from build123d import *

# Parameters (mm, degrees)
F1_START = 10
F0_R     = 79.5
F1_DEPTH = 5
F0_R_2   = 82
F2_DEPTH = 15
F0_R_3   = 87.5
F3_DEPTH = 4
F4_SIZE2 = 2.7474774195
F4_SIZE  = 1
F5_SIZE2 = 5.4949548389
F5_SIZE  = 2


with BuildPart() as f1:
    # F0 (on Top) → F1 (new body)
    with BuildSketch(Plane.XY.offset(F1_START)):
        Circle(F0_R)
    extrude(amount=F1_DEPTH)

    # F0 (on Top) → F2 (join)
    with BuildSketch(Plane.XY):
        Circle(F0_R_2)
        Circle(F0_R, mode=Mode.SUBTRACT)
    extrude(amount=F2_DEPTH)

    # F0 (on Top) → F3 (join)
    with BuildSketch(Plane.XY):
        Circle(F0_R_3)
        Circle(F0_R_2, mode=Mode.SUBTRACT)
    extrude(amount=F3_DEPTH)

    # F4
    f4_edges = [f1.edges().sort_by_distance(p)[0] for p in [
        (-82, 0, 15),
    ]]
    f4_side = f1.faces().sort_by_distance((0, 0, 15))[0]
    chamfer(f4_edges, length=F4_SIZE, length2=F4_SIZE2, reference=f4_side)

    # F5
    f5_edges = [f1.edges().sort_by_distance(p)[0] for p in [
        (-79.5, 0, 0),
    ]]
    f5_side = f1.faces().sort_by_distance((-81.974874, 0, 0))[0]
    chamfer(f5_edges, length=F5_SIZE, length2=F5_SIZE2, reference=f5_side)


solid = f1.part
Build history of the part. All positions in model axes, mm. A direction names the side the tool comes from. Round coordinates to 2 decimals unless told otherwise and drop trailing zeros. Write each loop counter-clockwise with the first axis right and the second up, starting at its lowest first coordinate (ties: lowest second). Pieces come first, ordered by that corner, then holes. Notation, with made-up numbers: M 85,82 L 101,82 A32 cw 101,110 Z; hole C 46.25,-4 d6. An arc over 180 degrees is marked long. Answer in a Markdown table with one row per item.
1. Which spindle directions (+Z, -Z, +X, -X, +Y, -Y) get a long thin tool onto all of the face, cutting with end or side? Do faces 5 (the face through (-78, -26, 4)), 6 (the face through (-72, 39, 0)), 7 (the face through (-1, 1, 10)). Say none if no direction does.
Geometry check:
| item | result |
|---|---|
| face 5 | +Z |
| face 6 | -Z, +X, -X, +Y, -Y |
| face 7 | -Z |
2. Saw through at A-A (y = 0). List the corners of the cut face in (x, z), and give its area (3 significant figures).
Geometry check:
| item | result |
|---|---|
| outline | M -87.5,0 L -81.5,0 L -79.5,5.49 L -79.5,10 L 79.5,10 L 79.5,5.49 L 81.5,0 L 87.5,0 L 87.5,4 L 82,4 L 82,12.25 L 81,15 L -81,15 L -82,12.25 L -82,4 L -87.5,4 Z |
| area | 900 mm2 |
3. Flat gauge pins, fed straight in: P1, Ø1, axis at x = 21.5, z = 11, coming from the +Y side; P2, Ø3, axis at x = 43, y = 25.5, coming from the -Z side; P3, Ø3, axis at y = 52.5, z = 12, coming from the +X side. Where does each tip first touch, or does it go through?
Geometry check:
| item | result |
|---|---|
| P1 | y = 79.27 |
| P2 | z = 10 |
| P3 | x = 64.21 |
4. Mould opens along Y. For faces 1 (the face through (-10.349, 78.823, 7.716)), 2 (the face through (-63.17, -48.43, 5.23)), 3 (the face through (77.32, 24.35, 14.83)), 4 (the face through (-1, 1, 15)) say: +Y half, -Y half, draft (parallel to the pull), parting line (faces both ways), or undercut.
Geometry check:
| item | result |
|---|---|
| face 1 | undercut |
| face 2 | undercut |
| face 3 | parting line |
| face 4 | draft |
5. Probe L1, parallel to Y at x = 0, z = 7.1; L2, parallel to Z at x = 71, y = -35; L3, parallel to Y at x = 36.5, z = 5.5. List the from-to ranges inside material, lowest first. Write a range as [from, to].
Geometry check:
| item | result |
|---|---|
| L1 | [-82, -79.5], [79.5, 82] |
| L2 | [10, 15] |
| L3 | [-73.43, -70.63], [70.63, 73.43] |
